Here's how the part is built. I have some questions about the finished solid (model axes, mm). Face numbers are marked on the shaded views. A direction names the side the tool comes from. Round coordinates to 2 decimals unless told otherwise and drop trailing zeros. Order: outer loops, then holes, each group sorted by start corner. A loop starts at its lowest first (then second) coordinate and runs counter-clockwise, first axis right, second up. Notation, with made-up numbers: (82, 66.5) -> (140, 66.5) arc R17 cw to (140, 90.5) -> close; hole circle Ø5 at (23, 75). An arc over 180 degrees is marked (long way). Answer in a Markdown table with one row per item.
```python
from build123d import *

# Parameters (mm, degrees)
SKETCH_1_R          = 1.6
SKETCH_1_R_2        = 3.2
EXTRUDE_1_DEPTH     = 4
SKETCH_2_R          = 1.525
EXTRUDE_2_DEPTH     = 10
CUT_EXTRUDE_1_DEPTH = 10
CUT_EXTRUDE_2_DEPTH = 10


with BuildPart() as part:
    # 草图1 → 凸台-拉伸1 (new body)
    with BuildSketch(Plane.XY):
        Polygon((0, 0), (0, 26), (10, 26), (18, 18), (18, 8), (10, 0), align=None)
        with Locations((5, 21)):
            Circle(SKETCH_1_R, mode=Mode.SUBTRACT)
        with Locations((5, 13)):
            Circle(SKETCH_1_R_2, mode=Mode.SUBTRACT)
        with Locations((5, 5)):
            Circle(SKETCH_1_R, mode=Mode.SUBTRACT)
        with Locations((13, 13)):
            Circle(SKETCH_1_R, mode=Mode.SUBTRACT)
    extrude(amount=EXTRUDE_1_DEPTH)

    # 草图2 → 凸台-拉伸2 (add)
    with BuildSketch(Plane.XY.offset(4)):
        with BuildLine():
            Line((13.468501969, 16.468501969), (16.5, 19.5))
            Line((16.5, 19.5), (11.5, 24.5))
            Line((11.5, 24.5), (8.468501969, 21.468501969))
            ThreePointArc((8.468501969, 21.468501969), (7.104490226, 18.203373302), (3.589329863, 17.796875))
            ThreePointArc((3.589329863, 17.796875), (0, 13), (3.589329863, 8.203125))
            ThreePointArc((3.589329863, 8.203125), (7.104490226, 7.796626698), (8.468501969, 4.531498031))
            Line((8.468501969, 4.531498031), (11.5, 1.5))
            Line((11.5, 1.5), (16.5, 6.5))
            Line((16.5, 6.5), (13.468501969, 9.531498031))
            ThreePointArc((13.468501969, 9.531498031), (9.5, 13), (13.468501969, 16.468501969))
        make_face()
        with Locations((5, 13)):
            Circle(SKETCH_2_R, mode=Mode.SUBTRACT)
    extrude(amount=EXTRUDE_2_DEPTH)

    # 草图3 → 切除-拉伸1 (cut)
    with BuildSketch(Plane(origin=(-1.5, 1.5, 0), x_dir=(0, 0, -1), z_dir=(0.7071067811865477, -0.7071067811865475, 0))):
        Polygon((-4, 25.455844123), (-14, 25.455844123), (-14, 21.168658492), align=None)
    extrude(amount=-CUT_EXTRUDE_1_DEPTH, mode=Mode.SUBTRACT)

    # 草图4 → 切除-拉伸2 (cut)
    with BuildSketch(Plane(origin=(11.5, 11.5, 0), x_dir=(0, 0, -1), z_dir=(0.7071067811865474, 0.7071067811865477, 0))):
        Polygon((-4, -7.071067812), (-14, -2.783882181), (-14, -7.071067812), align=None)
    extrude(amount=-CUT_EXTRUDE_2_DEPTH, mode=Mode.SUBTRACT)


solid = part.part
```
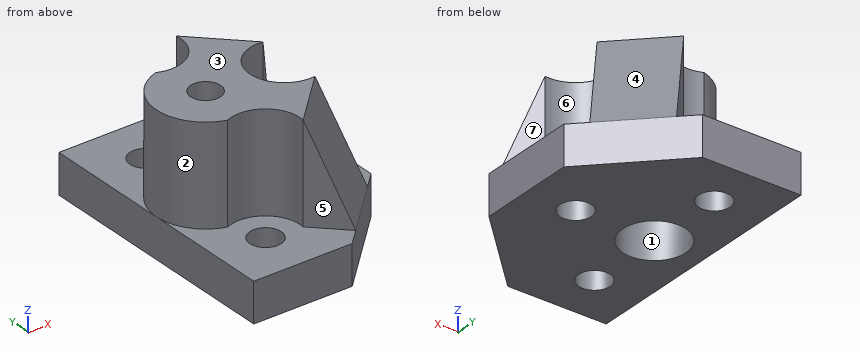
1. Suppose I cut it at B-B on x = 13. Write out the boundary of the cut face in (y, z), then the cut area to 3 significant figures.
Numbers:
| item | result |
|---|---|
| outline | (3, 0) -> (11.4, 0) -> (11.4, 4) -> (9.5, 4) -> (9.5, 14) -> (9.06, 14) -> (3, 4) -> close; (14.6, 0) -> (23, 0) -> (23, 4) -> (16.94, 14) -> (16.5, 14) -> (16.5, 4) -> (14.6, 4) -> close |
| area | 137 mm2 |
2. Suppose I cut it at A-A on x = 5. Write out the boundary of the cut face in (y, z) (3 decimals), then the cut area to 3 significant figures.
Numbers:
| item | result |
|---|---|
| outline | (0, 0) -> (3.4, 0) -> (3.4, 4) -> (0, 4) -> close; (6.6, 0) -> (9.8, 0) -> (9.8, 4) -> (11.475, 4) -> (11.475, 14) -> (8.5, 14) -> (8.5, 4) -> (6.6, 4) -> close; (14.525, 4) -> (16.2, 4) -> (16.2, 0) -> (19.4, 0) -> (19.4, 4) -> (17.5, 4) -> (17.5, 14) -> (14.525, 14) -> close; (22.6, 0) -> (26, 0) -> (26, 4) -> (22.6, 4) -> close |
| area | 112 mm2 |
3. Suppose I cut it at D-D on y = 20.5. Write out the boundary of the cut face in (x, z), then the cut area to 3 significant figures.
Numbers:
| item | result |
|---|---|
| outline | (0, 0) -> (3.48, 0) -> (3.48, 4) -> (0, 4) -> close; (6.52, 0) -> (15.5, 0) -> (15.5, 4) -> (9.44, 14) -> (8.46, 14) -> (8.46, 4) -> (6.52, 4) -> close |
| area | 89.9 mm2 |
4. For pin 1 Ø1 at (x, z) = (8, 5) entering from +Y; pin 2 Ø6 at (x, z) = (3, 12) entering from -Y; pin 3 Ø3.5 at (x, y) = (5, 13) entering from -Z; pin 4 Ø3 at (x, y) = (5, 5) entering from -Z, each with a flat end and sliding along its axis, tell me the tip position at first contact or that it passes through.
Numbers:
| item | result |
|---|---|
| pin 1 | stops at y = 21.5 |
| pin 2 | stops at y = 8.2 |
| pin 3 | stops at z = 4 |
| pin 4 | passes through |
5. Please list where these lines run through material, in increasing order: line 1 along Y through (x, z) = (5, 1.25); line 2 along Y through (x, z) = (6, 10.25); line 3 along X through (y, z) = (12, 8.25).
Numbers:
| item | result |
|---|---|
| line 1 | y = 0 to 3.4, 6.6 to 9.8, 16.2 to 19.4, 22.6 to 26 |
| line 2 | y = 8.35 to 11.85, 14.15 to 17.65 |
| line 3 | x = 0.1 to 3.85, 6.15 to 9.65 |
6. We'd pull the mould along X, two halves only. Please class the marked faces 1, 2, 3 and 4: released by +X, released by -X, zero draft, split by the parting line, or undercut.
Numbers:
| item | result |
|---|---|
| face 1 | undercut |
| face 2 | released by -X |
| face 3 | zero draft |
| face 4 | released by +X |
7. For the marked faces 5, 6 and 7, which set-ups out of +Z, -Z, +X, -X, +Y, -Y let a thin tool reach every point of the face, with its end or its side?
Numbers:
| item | result |
|---|---|
| face 5 | +Z, -X, -Y |
| face 6 | +Z |
| face 7 | +Z, +X |
